from build123d import *

# Parameters (mm, degrees)
BOSS_EXTRUDE1_DEPTH = 7.62


with BuildPart() as part:
    # Sketch1 → Boss-Extrude1 (new body)
    with BuildSketch(Plane.XY.offset(74.309059093)):
        Polygon((-16.83862503, 48.477236207), (-79.60202503, 52.922236207), (-79.60202503, 44.032236207), (-28.604506433, 16.328823125), (-61.627708465, 9.316547792), (-79.60202503, 5.499811409), (-79.60202503, -2.831388591), (-16.83862503, 9.937236207), (-16.83862503, 18.827236207), (-60.783589078, 42.699485785), (-28.604506433, 40.420513926), (-16.83862503, 39.587236207), align=None)
    extrude(amount=-BOSS_EXTRUDE1_DEPTH)


solid = part.part
Check sheet for the modelled part. Datum: model origin and axes. Units: mm. Give positions to 0.01 mm unless a question says otherwise; leave off trailing zeros. Write each loop counter-clockwise with the first axis right and the second up, starting at its lowest first coordinate (ties: lowest second). Pieces come first, ordered by that corner, then holes. Notation, with made-up numbers: (6, 76) -> (40, 76) arc R9 ccw to (40, 80) -> close; hole circle Ø6 at (-21.5, 82.5). An arc over 180 degrees is marked (long way). Use one line per item in the form item = value. Start each with the question number.
1. Section check A-A (x = -57.5). Record the cut outline in (y, z).
2. Thickness scan on line 1 along Y through (x, z) = (-57, 74.25); line 2 along Y through (x, z) = (-32, 74); line 3 along Y through (x, z) = (-25, 70.5). Record the ranges inside material, lowest first. Write a range as from..to.
3. Mould release check, pull along Y, two halves, no side actions. Record for faces 1 (the flat face through (-79.602, 49, 71)), 2 (the flat face through (-54.46, 30.374, 70.552)), 3 (the flat face through (-48.66, 3.464, 70.552)): pulls with the +Y half, pulls with the -Y half, needs draft (parallel to the pull), parting line crosses it, or undercut.
4. Section check D-D (x = -47). Record the cut outline in (y, z).
5. Section check C-C (x = -73). Record the cut outline in (y, z), and give its area (3 significant figures).
6. Section check B-B (z = 67.75). Record the cut outline in (x, y).
7. Go/stop test with flat-tipped pins: P1, Ø3, axis at x = -29, z = 68.5, coming from the -Y side; P2, Ø2, axis at x = -68, z = 68.5, coming from the -Y side. Record where each tip stops, or that it passes through.
Conclusion:
q1.outline = (1.67, 66.69) -> (10.19, 66.69) -> (10.19, 74.31) -> (1.67, 74.31) -> close; (32.03, 66.69) -> (40.92, 66.69) -> (40.92, 74.31) -> (32.03, 74.31) -> close; (42.47, 66.69) -> (51.36, 66.69) -> (51.36, 74.31) -> (42.47, 74.31) -> close
q2.line_1 = 1.77..10.3, 31.75..40.64, 42.43..51.32
q2.line_2 = 6.85..15.61, 18.17..27.06, 40.66..49.55
q2.line_3 = 8.28..23.26, 40.17..49.06
q3.face_1 = needs draft
q3.face_2 = undercut
q3.face_3 = pulls with the -Y half
q4.outline = (3.8, 66.69) -> (12.42, 66.69) -> (12.42, 74.31) -> (3.8, 74.31) -> close; (26.32, 66.69) -> (35.21, 66.69) -> (35.21, 74.31) -> (26.32, 74.31) -> close; (41.72, 66.69) -> (50.61, 66.69) -> (50.61, 74.31) -> (41.72, 74.31) -> close
q5.outline = (-1.49, 66.69) -> (6.9, 66.69) -> (6.9, 74.31) -> (-1.49, 74.31) -> close; (40.45, 66.69) -> (52.45, 66.69) -> (52.45, 74.31) -> (40.45, 74.31) -> close
q5.area = 155 mm²
q6.outline = (-79.6, -2.83) -> (-16.84, 9.94) -> (-16.84, 18.83) -> (-60.78, 42.7) -> (-16.84, 39.59) -> (-16.84, 48.48) -> (-79.6, 52.92) -> (-79.6, 44.03) -> (-28.6, 16.33) -> (-79.6, 5.5) -> close
q7.P1 = 7.16
q7.P2 = -0.67
